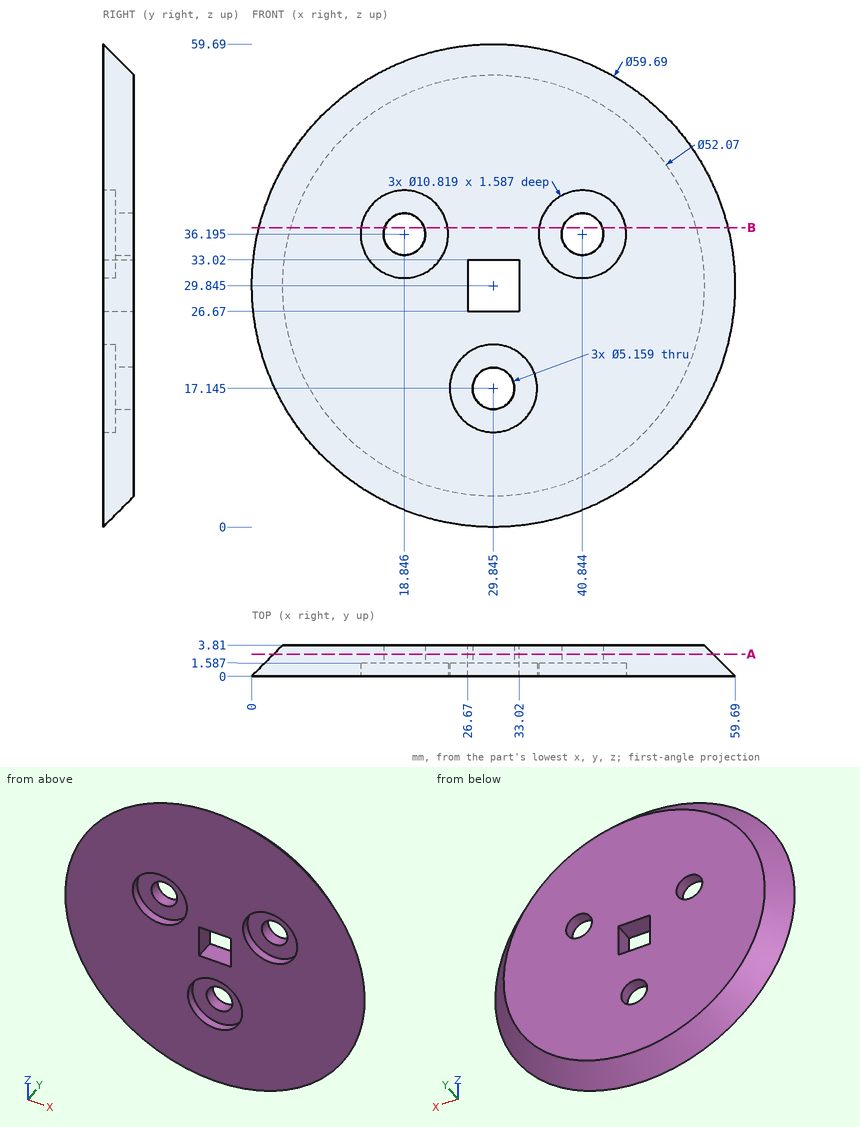
Answer from the drawing. Dimensions are ordinates in mm from the lowest x, y and z of the part. Give positions to 0.01 mm unless a question says otherwise; leave off trailing zeros. Write each loop counter-clockwise with the first axis right and the second up, starting at its lowest first coordinate (ties: lowest second). Pieces come first, ordered by that corner, then holes. Notation, with made-up numbers: (1.5, 6.25) -> (6.5, 6.25) arc R13 ccw to (6.5, 14.25) -> close; hole circle Ø8 at (-7.75, -19.75). An arc over 180 degrees is marked (long way). One line per question, with ' | ' between items. Start each with the question number.
1. Section B-B (z = 37) is taken. State how many separate pieces and enclosed holes the cut face has, plus the area to 3 significant figures.
2. Find the intervals of material crossed by probe 1 along Z at (x, y) = (27, 1.05) (1 decimal); probe 2 along X at (y, z) = (0.55, 33.5) (1 decimal); probe 3 along Y at (x, z) = (34, 15.5), in increasing order.
3. Section A-A (y = 2.7) is taken. Determine the outline of the cut face in (x, z) (1 decimal).
4. Given pin 1 Ø1.1 at (y, z) = (1.5, 30.5) entering from -X; pin 2 Ø8.5 at (x, z) = (29.845, 17.145) entering from -Y; pin 3 Ø4 at (x, z) = (40.84, 36.2) entering from +Y; pin 4 Ø1.9 at (x, y) = (31.5, 2.5) entering from -Z (1 decimal), each flat-ended and moving along its own axis, determine where each tip first touches the part or whether it passes through.
Response values:
1) separate pieces: 3 | enclosed holes: 0 | area: 150 mm2
2) probe 1: 1.2 to 12.5, 21.7 to 26.7, 33 to 58.5 | probe 2: 0.8 to 14.2, 23.5 to 36.2, 45.5 to 58.9 | probe 3: 1.59 to 3.81
3) outline: circle Ø54.3 at (29.8, 29.8); hole circle Ø5.2 at (18.8, 36.2); hole (26.7, 26.7) -> (33, 26.7) -> (33, 33) -> (26.7, 33) -> close; hole circle Ø5.2 at (29.8, 17.1); hole circle Ø5.2 at (40.8, 36.2)
4) pin 1: x = 0.96 | pin 2: y = 1.59 | pin 3: through | pin 4: z = 1.6
